from build123d import *

# Parameters (mm, degrees)
F2_DEPTH = 2
F3_DEPTH = 23
F5_DEPTH = 23


# Not quite as in the source:
# - a feature of the source that left no trace in its solid (it failed there, or was rolled back) is left out


with BuildPart() as f2:
    # F1 (on Top) → F2 (new body)
    with BuildSketch(Plane.XY):
        with BuildLine():
            ThreePointArc((37.2509612746, 50), (13.7972702688, 58.9420922887), (-10.4728523554, 52.5391410864))
            ThreePointArc((-10.4728523554, 52.5391410864), (-25.3288691863, 58.932170126), (-38.8117617996, 50))
            Line((-38.8117617996, 50), (-54.0782060256, 50))
            Line((-54.0782060256, 50), (-38.8004282479, -5))
            Line((-38.8004282479, -5), (38.8004282479, -5))
            Line((38.8004282479, -5), (54.0782060256, 50))
            Line((54.0782060256, 50), (37.2509612746, 50))
        make_face()
    extrude(amount=F2_DEPTH)

    # F0 (on Top) → F3 (join)
    with BuildSketch(Plane.XY):
        with BuildLine():
            Line((-35.4307118382, 45), (-47.5, 45))
            Line((-47.5, 45), (-35, 0))
            Line((-35, 0), (35, 0))
            Line((35, 0), (47.5, 45))
            Line((47.5, 45), (35.4307118382, 45))
            ThreePointArc((35.4307118382, 45), (11.6189500386, 54), (-12.192811761, 45))
            ThreePointArc((-12.192811761, 45), (-23.8117617996, 54), (-35.4307118382, 45))
        make_face()
    extrude(amount=F3_DEPTH)

    # F4 (on face) → F5 (cut, through all)
    with BuildSketch(Plane.XY.offset(23)):
        with BuildLine():
            ThreePointArc((35.3170512284, 44.7), (11.4242314878, 53.6994689692), (-12.3689964911, 44.4399020665))
            ThreePointArc((-12.3689964911, 44.4399020665), (-23.678456811, 53.6992405642), (-35.1959613762, 44.7))
            Line((-35.1959613762, 44.7), (-47.1053076385, 44.7))
            Line((-47.1053076385, 44.7), (-34.7719743051, 0.3))
            Line((-34.7719743051, 0.3), (34.7719743051, 0.3))
            Line((34.7719743051, 0.3), (47.1053076385, 44.7))
            Line((47.1053076385, 44.7), (35.3170512284, 44.7))
        make_face()
    extrude(amount=-F5_DEPTH, mode=Mode.SUBTRACT)


solid = f2.part
Input: part model. Units: mm. Frame: model coordinates. A direction names the side the tool comes from. Coordinates: 2 decimals unless noted, no trailing zeros. Loops run counter-clockwise (first coordinate to the right, second up) from the corner with the lowest first, then second, coordinate; pieces in that order, holes last. Notation, with made-up numbers: (-36.75, 61) -> (9.25, 61) arc R19 cw to (9.25, 81) -> close; hole circle Ø9 at (-13, 62.25). An arc over 180 degrees is marked (long way). Write item = value, one per line. Start each with the question number.
Item 1: Mould query, pull axis Y, two halves, no side actions, for faces 4 (the face through (42, 45, 12)), 5 (the face through (-12, 46, 0)), 6 (the face through (-41, 44.7, 12)), 7 (the face through (11.8, 53.7, 11.7)). Classes: pulls with the +Y half, pulls with the -Y half, needs draft (parallel to the pull), parting line crosses it, or undercut.
Item 2: Cut plane A-A, the plane z = 9.75. Return loops of the section in (x, y).
Item 3: Cut plane B-B, the plane x = -28.5. Return loops of the section in (y, z).
Item 4: First-contact query: P1, Ø13.5, axis at x = 42.5, z = 15.5, coming from the +Y side; P2, Ø0.6, axis at x = -50, z = 0.5, coming from the +Y side; P3, Ø2, axis at x = 15, z = 8.5, coming from the +Y side. Flat tips, straight axial feed; report the tip coordinate or a pass-through.
Item 5: Cut plane C-C, the plane y = 15. Return loops of the section in (x, z).
Item 6: Material intervals for line 1 (Z direction, x = -38, y = 8); line 2 (X direction, y = 38, z = 21); line 3 (Y direction, x = -13, z = 2.5), sorted ascending.
Item 7: Reachability of faces 1 (the face through (-41, 45, 12)), 2 (the face through (-46, 50, 1)), 3 (the face through (40.852, 22.189, 11.661)) from +Z, -Z, +X, -X, +Y, -Y: full face, straight path, thin tool, end or side. Return the list, or none.
Ans:
q1.face_4 = pulls with the +Y half
q1.face_5 = needs draft
q1.face_6 = undercut
q1.face_7 = undercut
q2.outline = (-47.5, 45) -> (-35, 0) -> (35, 0) -> (47.5, 45) -> (35.43, 45) arc R36 ccw to (-12.19, 45) arc R12 ccw to (-35.43, 45) -> close; hole (-47.11, 44.7) -> (-34.77, 0.3) -> (34.77, 0.3) -> (47.11, 44.7) -> (35.32, 44.7) arc R35.7 ccw to (-12.37, 44.44) arc R11.7 ccw to (-35.2, 44.7) -> close
q3.outline = (-5, 0) -> (0.3, 0) -> (0.3, 23) -> (0, 23) -> (0, 2) -> (-5, 2) -> close; (52.72, 0) -> (58.34, 0) -> (58.34, 2) -> (53.05, 2) -> (53.05, 23) -> (52.72, 23) -> close
q4.P1 = 45
q4.P2 = 50
q4.P3 = 53.92
q5.outline = (-44.36, 0) -> (-38.86, 0) -> (-38.86, 23) -> (-39.17, 23) -> (-39.17, 2) -> (-44.36, 2) -> close; (38.86, 0) -> (44.36, 0) -> (44.36, 2) -> (39.17, 2) -> (39.17, 23) -> (38.86, 23) -> close
q6.line_1 = 0 to 2
q6.line_2 = -45.56 to -45.24, 45.24 to 45.56
q6.line_3 = 0 to 0.3, 46.47 to 47.21
q7.face_1 = +Z, -X, +Y
q7.face_2 = +Z, -Z, -X, +Y
q7.face_3 = +Z, -Z
